Part model, mm, in its own coordinate system. A direction names the side the tool comes from. Give positions to 0.01 mm unless a question says otherwise; leave off trailing zeros. Order: outer loops, then holes, each group sorted by start corner. A loop starts at its lowest first (then second) coordinate and runs counter-clockwise, first axis right, second up.
1. Slice it at D-D on x = -17. List the corners of the cut face in (y, z).
2. Probe line 1 (Z direction, x = -3.5, y = -0.15); line 2 (Y direction, x = -16.5, z = 2); line 3 (Z direction, x = -25, y = 1.2). List the from-to ranges inside material, lowest first.
3. Slice it at C-C on x = -3. List the corners of the cut face in (y, z).
4. Which spindle directions (+Z, -Z, +X, -X, +Y, -Y) get a long thin tool onto all of the face, cutting with end or side? Do faces 1 (the cylindrical face through (-19.93, 0.54, -2.44)), 2 (the flat face through (0, 0, 0)), 3 (the flat face through (-25, 0, 2)). Say none if no direction does.
5. Drop flat-ended pins along their axis: pin 1 Ø0.6 at (y, z) = (-0.5, 2.5) entering from -X; pin 2 Ø1.5 at (x, z) = (-25.5, -0.5) entering from +Y; pin 3 Ø3.5 at (x, y) = (-25.5, 0.5) entering from +Z. Give the stop position or say it passes through.
6. Slice it at B-B on z = 0. List the corners of the cut face in (x, y).
7. Slice it at A-A on y = 0. List the corners of the cut face in (x, z).
Solid Edge part; units mm, degrees
sketch "Sketch1" plane through (0, 0, 0) normal (1, 0, 0) x (0, 1, 0)
  circle A0 centre (0, 0) radius 3
extrude "Protrusion1" add sketch "Sketch1" against normal blind 30.3
sketch "Sketch2" plane through (-30.3, 0, 0) normal (-1, 0, 0) x (0, -1, 0)
  circle A0 centre (0, 0) radius 2.5
extrude "Extrusionsausschnitt_1" cut sketch "Sketch2" against normal blind 20 flip side to cut
fillet "Verrundung_2" radius 1 1 edges at (-30.3, 2.5, 0)
fillet "Verrundung_3" radius 1 1 edges at (-10.3, 3, 0)
sketch "Sketch3" plane through (-30.3, 0, 0) normal (-1, 0, 0) x (0, -1, 0)
  line L0 (-1.5, 2) -> (1.5, 2)
extrude "Extrusionsausschnitt_3" cut sketch "Sketch3" against normal blind 10 material side at (-30.3, 0, 2.05)
properties material "Aluminium, 1060"
Data:
1. outline: circle Ø5 at (0, 0)
2. line 1: z = -3 to 3
2. line 2: y = -1.5 to 1.5
2. line 3: z = -2.19 to 2
3. outline: circle Ø6 at (0, 0)
4. face 1: -X
4. face 2: +Z, -Z, +X, +Y, -Y
4. face 3: +Z, -X, +Y, -Y
5. pin 1: stops at x = -20.3
5. pin 2: stops at y = 2.5
5. pin 3: stops at z = 2
6. outline: (-30.3, -1.5) arc R1 ccw to (-29.3, -2.5) - (-10.3, -2.5) arc R1 ccw to (-9.43, -3) - (0, -3) - (0, 3) - (-9.43, 3) arc R1 ccw to (-10.3, 2.5) - (-29.3, 2.5) arc R1 ccw to (-30.3, 1.5) - close
7. outline: (-30.3, -1.5) arc R1 ccw to (-29.3, -2.5) - (-10.3, -2.5) arc R1 ccw to (-9.43, -3) - (0, -3) - (0, 3) - (-9.43, 3) arc R1 ccw to (-10.3, 2.5) - (-20.3, 2.5) - (-20.3, 2) - (-30.17, 2) arc R1 ccw to (-30.3, 1.5) - close
